Autodesk Fusion 360 part; units mm, degrees
sketch "スケッチ1" plane through (0, 0, 0) normal (0, 0, 1) x (1, 0, 0)
  circle A0 centre (0, 0) radius 2.65
  line L0 (0, -7.5) -> (0, 7.5)
  line L1 (0, 7.5) -> (-6.3, 7.5)
  line L2 (-6.3, 7.5) -> (-6.3, -7.5)
  line L3 (-6.3, -7.5) -> (0, -7.5)
  line L4 (0, -7.5) -> (0, 7.5)
  arc A1 (0, -7.5) -> (0, 7.5) centre (0, 0) ccw
  line L5 (2.65, 0) -> (-2.65, 0)
  line L6 (3.8, 1.15) -> (1.5, 1.15)
  line L7 (1.5, 1.15) -> (1.5, -1.15)
  line L8 (1.5, -1.15) -> (3.8, -1.15)
  line L9 (3.8, -1.15) -> (3.8, 1.15)
  line L10 (3.8, 1.15) -> (1.5, -1.15) construction
  line L11 (1.5, 1.15) -> (3.8, -1.15) construction
  point P0 (2.65, 0)
  dimension "d1" = 5.3
  dimension "d2" = 15
  dimension "d5" = 6.3
  dimension "d6" = 15
  dimension "d31" = 2.3
  dimension "d32" = 2.3
extrude "押し出し1" add sketch "スケッチ1" along normal blind 1 contours A0 L0 L4 A1 L6 L8 L9 | A0 L0 L1 L2 L3 L4
sketch "スケッチ2" plane through (-6.3, 0, 0) normal (-1, 0, 0) x (0, -1, 0)
  line L0 (-7.5, 0) -> (7.5, 0)
  line L1 (7.5, 0) -> (7.5, 1)
  line L2 (7.5, 1) -> (-7.5, 1)
  line L3 (-7.5, 1) -> (-7.5, 0)
  line L4 (-7.5, 1) -> (-7.5, 16) construction
  line L5 (7.5, 1) -> (7.5, 16) construction
  line L6 (-7.5, 1) -> (-7.5, 1.7604)
  line L7 (-6.5, 1) -> (-7.5, 1)
  line L8 (-7.5, 1) -> (-7.5, 1.7604)
  line L9 (-4.7298, 1.4909) -> (7.5, 4.8825)
  line L10 (-4.663, 1) -> (10.2045, 1) construction
  line L11 (-7.5, 1.7604) -> (5.6313, 5.4021)
  line L12 (5.6313, 5.8839) -> (-7.5, 9.5255)
  line L13 (-5.6313, 10.045) -> (7.5, 6.4034)
  line L14 (7.5, 6.4034) -> (7.5, 4.8825)
  line L15 (-5.6313, 10.5268) -> (7.5, 14.1685)
  line L16 (-7.5, 11.0463) -> (3.758, 14.1685)
  line L17 (-7.5, 11.0463) -> (-7.5, 9.5255)
  line L18 (7.5, 14.1685) -> (3.758, 14.1685)
  arc A0 (-4.7298, 1.4909) -> (-4.663, 1) centre (-4.663, 1.25) ccw
  arc A1 (5.6313, 5.4021) -> (5.6313, 5.8839) centre (5.5645, 5.643) ccw
  arc A2 (-5.6313, 10.5268) -> (-5.6313, 10.045) centre (-5.5645, 10.2859) ccw
  point P0 (6.5, 5.643)
  point P1 (-6.5, 10.2859)
  dimension "d7" = 15
  dimension "d8" = 15
  dimension "d9" = 15.5
  dimension "d15" = 15.5
  dimension "d16" = 1
  dimension "d17" = 1
  dimension "d18" = 15.5
  dimension "d19" = 15.5
  dimension "d20" = 1
  dimension "d21" = 1
  dimension "d22" = 15.5
  dimension "d23" = 15.5
  dimension "d24" = 1
  dimension "d25" = 1
  dimension "d26" = 0.25
  dimension "d27" = 0.25
  dimension "d28" = 0.25
extrude "押し出し2" add sketch "スケッチ2" against normal blind 3.5 contours L2 L6 L7 L8 L9 L11 L12 L13 L14 L15 L16 L17 L18 A0 A1 A2
sketch "スケッチ3" plane through (0, 0, 14.1685) normal (0, 0, 1) x (-1, 0, 0)
  line L0 (6.3, 3.758) -> (6.3, 7.5)
  line L1 (6.3, 7.5) -> (2.8, 7.5)
  line L2 (2.8, 7.5) -> (2.8, 3.758)
  line L3 (2.8, 3.758) -> (6.3, 3.758)
  line L4 (2.8, -4.663) -> (6.3, -4.663)
  line L5 (6.3, -4.663) -> (6.3, 7.5)
  line L6 (6.3, 7.5) -> (0, 7.5)
  arc A0 (0, 7.5) -> (0, -7.5) centre (0, 0) ccw
  line L7 (0, -7.5) -> (2.8, -7.5)
  line L8 (2.8, -7.5) -> (2.8, -4.663)
  line L9 (-3.8, -1.15) -> (-3.8, 1.15)
  line L10 (-3.8, 1.15) -> (-2.3875, 1.15)
  arc A1 (-2.3875, -1.15) -> (-2.3875, 1.15) centre (0, 0) ccw
  line L11 (-2.3875, -1.15) -> (-3.8, -1.15)
  line L12 (6.3, -7.5) -> (6.3, 3.758)
  line L13 (6.3, 3.758) -> (2.8, 3.758)
  line L14 (2.8, 3.758) -> (2.8, -7.5)
  line L15 (2.8, -7.5) -> (6.3, -7.5)
  line L16 (6.3, 5) -> (6.3, -5)
  line L17 (-7.5, 0) -> (-7.5, -7.5)
  line L18 (-7.5, -7.5) -> (6.3, -7.5)
  line L19 (6.3, -4.663) -> (6.3, -7.5)
  line L20 (6.3, -5) -> (-7.5, -5)
  line L21 (-20, 0) -> (-2.5, 0)
  line L22 (6.3, 5) -> (-7.5, 5)
  line L23 (-7.5, 0) -> (-7.5, 7.5)
  line L24 (6.3, 4.663) -> (6.3, 7.5)
  line L25 (-7.5, 7.5) -> (6.3, 7.5)
  point P0 (6.3, 0)
  dimension "d38" = 5
extrude "押し出し3" add sketch "スケッチ3" along normal blind 1 contours L0 L2 L3 L5 L13 L16 L22 L24 | L3 L4 L5 L12 L13 L14 L16 | L4 L8 L12 L14 L16 L19 L20 | L0 L1 L2 L5 L6 L22 L24 L25 | L2 L6 A0 L22 L25 | L8 L12 L14 L15 L18 L19 L20 | A0 L22 L23 L25 | A0 L7 L8 L14 L18 L20 | A0 L17 L18 L20
equation "d5 = d1 + 1 mm"
equation "d6 = d2"
equation "d8 = d7"
equation "d15 = d9"
equation "d17 = d16"
equation "d18 = d9"
equation "d19 = d9"
equation "d20 = d16"
equation "d21 = d16"
equation "d22 = d9"
equation "d23 = d9"
equation "d24 = d16"
equation "d25 = d16"
equation "d31 = d32"
Here's how the part is built. I have some questions about the finished solid (model axes, mm). A direction names the side the tool comes from. Give positions to 0.01 mm unless a question says otherwise; leave off trailing zeros. Write each loop counter-clockwise with the first axis right and the second up, starting at its lowest first coordinate (ties: lowest second). Pieces come first, ordered by that corner, then holes.
(1) Will these pins go through, and if not, where does the flat tip stop? pin 1 (4.5 mm diameter, centred on y = 3, z = 9.5, fed in from +X); pin 2 (1.5 mm diameter, centred on x = 0, y = 3.5, fed in from +Z); pin 3 (0.8 mm diameter, centred on x = 3, z = 0.5, fed in from +Y).
Output values:
pin 1: stops at x = -2.8
pin 2: stops at z = 1
pin 3: stops at y = 7.03
(2) On a 3-axis mill with a long thin cutter (end or side, diameter ignored), from which of +Z, -Z, +X, -X, +Y, -Y can I reach the whole of each face in a straight line? I mean faces 4 (the face through (2, 5, 15)), 5 (the face through (-4.57, 0.84, 7.68)), 6 (the face through (2, 2, 1)), 7 (the face through (2, -6, 14.168)). Say none if no direction works.
Output values:
face 4: +Z, +X
face 5: +X, -X, +Y
face 6: +X, -Y
face 7: +X, +Y, -Y
(3) If I drill on L1, parallel to X at y = 0, z = 0.5; L2, parallel to Z at x = 1.5, y = 5.25; L3, parallel to Y at x = 0, z = 0.7, over which ranges is the centre line in solid material (lowest first)?
Output values:
L1: x = -6.3 to -2.65, 3.8 to 7.5
L2: z = 0 to 1, 14.17 to 15.17
L3: y = -7.5 to -2.65, 2.65 to 7.5
(4) Imagine slicing it at B-B, the plane y = 6.75. Write out the boundary of the cut face in (x, z).
Output values:
outline: (-6.3, 0) - (3.27, 0) - (3.27, 1) - (-2.8, 1) - (-2.8, 1.97) - (-6.3, 1.97) - close; (-6.3, 9.32) - (-2.8, 9.32) - (-2.8, 11.25) - (-6.3, 11.25) - close; (-6.3, 14.17) - (7.5, 14.17) - (7.5, 15.17) - (-6.3, 15.17) - close
(5) Imagine slicing it at C-C, the plane y = -2.25. Write out the boundary of the cut face in (x, z), and give its area (3 significant figures).
Output values:
outline: (-6.3, 0) - (-1.4, 0) - (-1.4, 1) - (-6.3, 1) - close; (-6.3, 3.43) - (-2.8, 3.43) - (-2.8, 4.46) - (-6.3, 4.46) - close; (-6.3, 6.82) - (-2.8, 6.82) - (-2.8, 7.86) - (-6.3, 7.86) - close; (-6.3, 12.71) - (-2.8, 12.71) - (-2.8, 13.75) - (-6.3, 13.75) - close; (-6.3, 14.17) - (-2.8, 14.17) - (-2.8, 15.17) - (-6.3, 15.17) - close; (1.4, 0) - (7.15, 0) - (7.15, 1) - (1.4, 1) - close
area: 25.1 mm2
(6) Thinking about a two-plate mould opening in Y: for faces 1 (the face through (3.8, 0, 0.5)), 2 (the face through (-5, 7.5, 10)), 3 (the face through (7.5, 0.16, 0.49)), which applies, pulls with the +Y half, pulls with the -Y half, needs draft (parallel to the pull), parting line crosses it, or undercut?
Output values:
face 1: undercut
face 2: pulls with the +Y half
face 3: parting line crosses it
(7) Imagine slicing it at D-D, the plane z = 8.5. Write out the boundary of the cut face in (x, y).
Output values:
outline: (-6.3, 0.06) - (-2.8, 0.06) - (-2.8, 3.8) - (-6.3, 3.8) - close
(8) Imagine slicing it at A-A, the plane y = 1.5. Write out the boundary of the cut face in (x, z), and give its area (3 significant figures).
Output values:
outline: (-6.3, 0) - (-2.18, 0) - (-2.18, 1) - (-6.3, 1) - close; (-6.3, 2.39) - (-2.8, 2.39) - (-2.8, 3.42) - (-6.3, 3.42) - close; (-6.3, 7.86) - (-2.8, 7.86) - (-2.8, 8.9) - (-6.3, 8.9) - close; (-6.3, 11.67) - (-2.8, 11.67) - (-2.8, 12.71) - (-6.3, 12.71) - close; (-6.3, 14.17) - (-2.8, 14.17) - (-2.8, 15.17) - (-6.3, 15.17) - close; (2.18, 0) - (7.35, 0) - (7.35, 1) - (2.18, 1) - close
area: 23.7 mm2
